Input: part model. Units: mm. Frame: model coordinates. A direction names the side the tool comes from. Coordinates: 2 decimals unless noted, no trailing zeros. Loops run counter-clockwise (first coordinate to the right, second up) from the corner with the lowest first, then second, coordinate; pieces in that order, holes last.
Item 1: Section A-A on z = 74. Return loops of the section in (x, y).
Item 2: Contact query for flat-ended pins moving along their axis: P1, Ø4.5, axis at x = 0.5, y = 3, coming from the +Z side; P2, Ø5, axis at x = 42, y = 14, coming from the -Z side; P3, Ø1.5, axis at y = 0, z = 133.5, coming from the +X side; P4, Ø2, axis at x = 10, z = 87, coming from the -Y side. Output: stop coordinate, or through.
Item 3: Pull-direction query (X, two-part tool) for faces 3 (the cylindrical face through (-2.17, -9.76, 79.02)), 4 (the flat face through (-5, 4, 0)), 5 (the cylindrical face through (-7.493, 0.33, 76.485)); classes: released by +X, released by -X, zero draft, split by the parting line, or undercut.
Item 4: Ray query, line 1 along X through (y, z) = (0, 37); line 2 along Z through (x, y) = (-20.5, -7). Return the intervals inside material, ascending.
Item 5: Reachability of faces 1 (the flat face through (4, 7, 150)), 2 (the flat face through (0, 0, 5)) from +Z, -Z, +X, -X, +Y, -Y: full face, straight path, thin tool, end or side. Return the list, or none.
```python
from build123d import *

# Parameters (mm, degrees)
F1_R     = 10
F2_DEPTH = 150
F3_T     = -2.5
F4_DEPTH = 5
F5_R     = 4.999


# Not quite as in the source:
# - a fillet or chamfer is up to 0.001 mm smaller than in the source, because OpenCascade refuses the exact size


with BuildPart() as f2:
    # F1 (on Top) → F2 (new body)
    with BuildSketch(Plane.XY):
        Circle(F1_R)
    extrude(amount=F2_DEPTH)

    # F3
    f3_openings = [f2.faces().sort_by_distance(p)[0] for p in [
        (0, 0, 150),
    ]]
    offset(amount=F3_T, openings=f3_openings)

    # F0 (on Top) → F4 (join)
    with BuildSketch(Plane.XY):
        with BuildLine():
            add(Edge.make_bspline(
                [(75, 0), (75, 51.9615242271), (-37.5, 25.9807621135), (-150, 0), (-37.5, -25.9807621135), (75, -51.9615242271), (75, 0)],
                knots=[0, 0, 0, 2.0943951024, 2.0943951024, 4.1887902048, 4.1887902048, 6.2831853072, 6.2831853072, 6.2831853072], degree=2, weights=[1, 0.5, 1, 0.5, 1, 0.5, 1]))
        make_face()
    extrude(amount=F4_DEPTH)

    # F5 (radius 5 in the source; OpenCascade refuses exactly that, so slightly less here)
    f5_edges = [f2.edges().sort_by_distance(p)[0] for p in [
        (-10, 0, 5),
        (-75, 9.6e-05, 5),
    ]]
    fillet(f5_edges, radius=F5_R)


solid = f2.part
```
Results found:
1. outline: circle Ø20 at (0, 0); hole circle Ø15 at (0, 0)
2. P1: stops at z = 5
2. P2: stops at z = 0
2. P3: stops at x = 10
2. P4: stops at y = -4.36
3. face 3: split by the parting line
3. face 4: zero draft
3. face 5: undercut
4. line 1: x = -10 to -7.5, 7.5 to 10
4. line 2: z = 0 to 5
5. face 1: +Z, +X, -X, +Y, -Y
5. face 2: +Z
